Source: CAD feature listing. Evaluate the final solid. Frame: model axes, mm. A direction names the side the tool comes from. Coordinates: 2 decimals unless noted, no trailing zeros. Order: outer loops, then holes, each group sorted by start corner. A loop starts at its lowest first (then second) coordinate and runs counter-clockwise, first axis right, second up.
```python
from build123d import *

# Parameters (mm, degrees)
SKETCH1_W           = 20
SKETCH1_H           = 20
SKETCH1_W_2         = 17
SKETCH1_H_2         = 17
BOSS_EXTRUDE1_DEPTH = 775.4
CUT_EXTRUDE1_DEPTH  = 5
SKETCH3_R           = 2.5
CUT_EXTRUDE8_DEPTH  = 5
CUT_EXTRUDE10_DEPTH = 101


with BuildPart() as part:
    # Sketch1 → Boss-Extrude1 (new body)
    with BuildSketch(Plane(origin=(0, 0, 0), x_dir=(1, 0, 0), z_dir=(0, 1, 0))):
        Rectangle(SKETCH1_W, SKETCH1_H)
        Rectangle(SKETCH1_W_2, SKETCH1_H_2, mode=Mode.SUBTRACT)
    extrude(amount=BOSS_EXTRUDE1_DEPTH)

    # Sketch2 → Cut-Extrude1 (cut)
    with BuildSketch(Plane.XY.offset(10)):
        with BuildLine():
            Line((-2.5, 766.9), (-2.5, 763.9))
            ThreePointArc((-2.5, 763.9), (0, 761.4), (2.5, 763.9))
            Line((2.5, 763.9), (2.5, 766.9))
            ThreePointArc((2.5, 766.9), (0, 769.4), (-2.5, 766.9))
        make_face()
    extrude(amount=-CUT_EXTRUDE1_DEPTH, mode=Mode.SUBTRACT)

    # Sketch3 → Cut-Extrude8 (cut)
    with BuildSketch(Plane.XY.offset(10)):
        with Locations((0, 723.9)):
            Circle(SKETCH3_R)
        with Locations((0, 681.9)):
            Circle(SKETCH3_R)
        with Locations((0, 583.1)):
            Circle(SKETCH3_R)
        with Locations((0, 541.1)):
            Circle(SKETCH3_R)
        with Locations((0, 442.3)):
            Circle(SKETCH3_R)
        with Locations((0, 400.3)):
            Circle(SKETCH3_R)
    extrude(amount=-CUT_EXTRUDE8_DEPTH, mode=Mode.SUBTRACT)

    # Sketch10 → Cut-Extrude10 (cut)
    with BuildSketch(Plane.ZY.offset(10)):
        with BuildLine():
            Line((-2.5, 766.9), (-2.5, 763.9))
            ThreePointArc((-2.5, 763.9), (0, 761.4), (2.5, 763.9))
            Line((2.5, 763.9), (2.5, 766.9))
            ThreePointArc((2.5, 766.9), (0, 769.4), (-2.5, 766.9))
        make_face()
    extrude(amount=-CUT_EXTRUDE10_DEPTH, mode=Mode.SUBTRACT)


solid = part.part
```
1. Section query A-A on z = -5.5. Return loops of the section in (x, y), plus the area to 3 significant figures.
Findings:
outline: (-10, 0) - (-8.5, 0) - (-8.5, 775.4) - (-10, 775.4) - close; (8.5, 0) - (10, 0) - (10, 775.4) - (8.5, 775.4) - close
area: 2,330 mm2
2. Access query for faces 1 (the face through (0, 382, 10)), 2 (the face through (0, 382, 8.5)). Directions: +Z, -Z, +X, -X, +Y, -Y. A direction counts if a zero-diameter tool reaches every point of the face in a straight line with its end or side. Return the directions, or none.
Findings:
face 1: +Z, +X, -X, +Y, -Y
face 2: +Y, -Y
3. Pin query (flat end, axial travel): P1, Ø3, axis at x = 0, y = 583.1, coming from the +Z side. Return the tip coordinate at first contact, or that it passes through.
Findings:
P1: stops at z = -8.5
4. Draft query along X for faces 3 (the face through (-8.5, 382, 0)), 4 (the face through (10, 382, 0)), 5 (the face through (-9, 0, 0)). Return one class per face: released by +X, released by -X, zero draft, split by the parting line, or undercut.
Findings:
face 3: undercut
face 4: released by +X
face 5: zero draft
5. Section query B-B on y = 51. Return loops of the section in (x, z), plus the area to 3 significant figures.
Findings:
outline: (-10, -10) - (10, -10) - (10, 10) - (-10, 10) - close; hole (-8.5, -8.5) - (8.5, -8.5) - (8.5, 8.5) - (-8.5, 8.5) - close
area: 111 mm2
6. Ray query, line 1 (X direction, y = 483, z = -4.5); line 2 (X direction, y = 681.9, z = 9.2). Return the intervals inside material, ascending.
Findings:
line 1: x = -10 to -8.5, 8.5 to 10
line 2: x = -10 to -2.5, 2.5 to 10
